Part print with two shaded views. Sizes in mm from the minimum x, y, z corner. A direction names the side the tool comes from. Give positions to 0.01 mm unless a question says otherwise; leave off trailing zeros. Order: outer loops, then holes, each group sorted by start corner. A loop starts at its lowest first (then second) coordinate and runs counter-clockwise, first axis right, second up. Notation, with made-up numbers: M -2,74 L 49,74 A11 ccw 49,82 Z; hole C -10,82.5 d2. An arc over 180 degrees is marked long. Return JSON: item names as keys, results as strings. Group by question number.
1. Pin check, flat tips, straight feed: pin 1 (4 mm diameter, centred on y = 12, z = 11.5, fed in from -X); pin 2 (1 mm diameter, centred on x = 21.5, z = 7, fed in from +Y); pin 3 (12 mm diameter, centred on x = 14.5, z = 15, fed in from +Y); pin 4 (2 mm diameter, centred on y = 11.5, z = 15, fed in from -X). Stop position of each tip, or through.
2. Two-plate mould, pull along X, no slides. Class the marked faces 5, 6 and 7: released by +X, released by -X, zero draft, split by the parting line, or undercut.
3. Wall check: probe 1 along Y at (x, z) = (12.5, 1.1); probe 2 along Z at (x, y) = (16.5, 1.75); probe 3 along Z at (x, y) = (9, 4.25). Give the ranges that are in metal, low to high. Write a range as [from, to].
4. 3-axis set-ups, long thin cutter, end or side, ignore diameter. For the marked faces 1, 2, 3 and 4: which of +Z, -Z, +X, -X, +Y, -Y reach the whole face in a straight line?
5. Slice it at B-B on x = 11.75. List the corners of the cut face in (y, z) (1 decimal), then the cut area to 3 significant figures.
6. Slice it at D-D on y = 15.5. List the corners of the cut face in (x, z) (1 decimal), then the cut area to 3 significant figures.
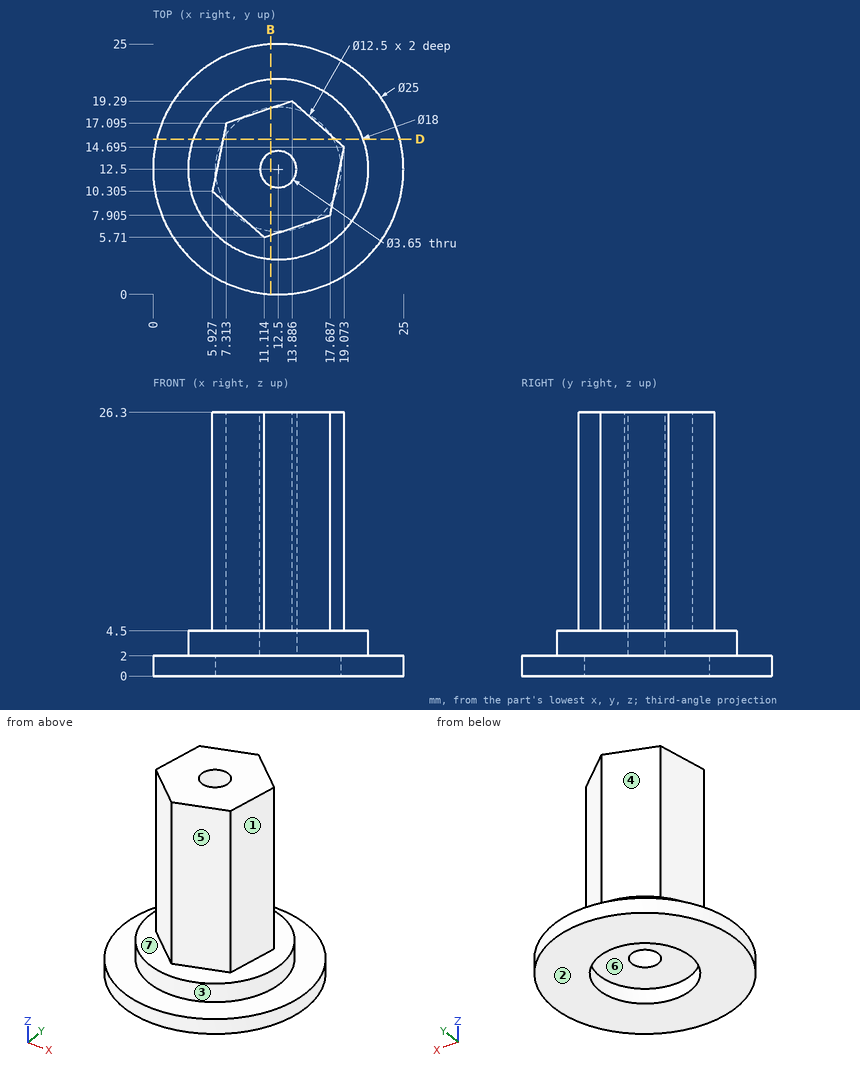
Result:
{
 "1": {"pin 1": "stops at x = 5.93", "pin 2": "passes through", "pin 3": "stops at y = 19.29", "pin 4": "stops at x = 5.97"},
 "2": {"face 5": "released by +X", "face 6": "undercut", "face 7": "zero draft"},
 "3": {"probe 1": "y = [0, 6.25], [18.75, 25]", "probe 2": "z = [0, 2]", "probe 3": "z = [0, 4.5]"},
 "4": {"face 1": "+Z, +X, -Y", "face 2": "-Z, +X, -X, +Y, -Y", "face 3": "+Z", "face 4": "+Z, -X, +Y"},
 "5": {"outline": "M 0,0 L 6.3,0 L 6.3,2 L 10.8,2 L 10.8,26.3 L 5.9,26.3 L 5.9,4.5 L 3.5,4.5 L 3.5,2 L 0,2 Z; M 14.2,2 L 18.7,2 L 18.7,0 L 25,0 L 25,2 L 21.5,2 L 21.5,4.5 L 18.6,4.5 L 18.6,26.3 L 14.2,26.3 Z", "area": "265 mm2"},
 "6": {"outline": "M 0.4,0 L 7,0 L 7,2 L 18,2 L 18,0 L 24.6,0 L 24.6,2 L 21,2 L 21,4.5 L 18.2,4.5 L 18.2,26.3 L 7,26.3 L 7,4.5 L 4,4.5 L 4,2 L 0.4,2 Z", "area": "313 mm2"}
}
